Here's how the part is built. I have some questions about the finished solid (model axes, mm). Face numbers are marked on the shaded views. A direction names the side the tool comes from. Coordinates: 2 decimals unless noted, no trailing zeros. Write each loop counter-clockwise with the first axis right and the second up, starting at its lowest first coordinate (ties: lowest second). Pieces come first, ordered by that corner, then holes. Notation, with made-up numbers: (-12, 12) -> (25, 12) arc R20 cw to (25, 28) -> close; hole circle Ø9 at (58.25, 53.5). An arc over 180 degrees is marked (long way). Answer in a Markdown table with one row per item. Add a question column.
Autodesk Inventor part; units mm, degrees
ref_plane "YZ Plane" through (0, 0, 0) normal (1, 0, 0) x (0, 1, 0)
ref_plane "XZ Plane" through (0, 0, 0) normal (0, 1, 0) x (-1, 0, 0)
ref_plane "XY Plane" through (0, 0, 0) normal (0, 0, 1) x (1, 0, 0)
sketch "スケッチ1" plane through (0, 0, 0) normal (0, 0, 1) x (1, 0, 0)
  line L0 (-25, 25) -> (25, 25)
  line L1 (25, 25) -> (25, -25)
  line L2 (25, -25) -> (-25, -25)
  line L3 (-25, -25) -> (-25, 25)
  line L4 (-23, 23) -> (23, 23)
  line L5 (23, 23) -> (23, -23)
  line L6 (23, -23) -> (-23, -23)
  line L7 (-23, -23) -> (-23, 23)
  point P0 (0, 0)
  dimension "d0" = 50
  dimension "d1" = 50
  dimension "d4" = 25
  dimension "d5" = 25
  dimension "d6" = 46
  dimension "d7" = 2
  dimension "d8" = 46
  dimension "d9" = 2
extrude "押し出し1" add sketch "スケッチ1" along normal blind 50
sketch "スケッチ2" plane through (25, -25, 0) normal (1, 0, 0) x (0, 0, -1)
  line L0 (-50, 50) -> (-50, 0)
  line L1 (0, 0) -> (-50, 0)
  line L2 (-50, 20) -> (-13.5, 20)
  line L3 (-13.5, 7) -> (-50, 7)
  line L4 (-50, 7) -> (-50, 20)
  arc A0 (-13.5, 7) -> (-13.5, 20) centre (-13.5, 13.5) ccw
  point P0 (0, 25)
  point P1 (-7, 13.5)
  dimension "d34" = 13
  dimension "d35" = 7
  dimension "d43" = 13
  dimension "d44" = 6.5
  dimension "d46" = 36.5
extrude "押し出し2" cut sketch "スケッチ2" against normal blind 30.5
sketch "スケッチ3" plane through (25, -25, 0) normal (1, 0, 0) x (0, 0, -1)
  arc A0 (-13.5, 7) -> (-13.5, 20) centre (-13.5, 13.5) ccw
  line L0 (-13.5, 7) -> (-50, 7)
  circle A1 centre (-7, 21.5) radius 1
  circle A2 centre (-43, 21.5) radius 1
  circle A3 centre (-43, 5.5) radius 1
  circle A4 centre (-7, 5.5) radius 1
  point P0 (0, 25)
  dimension "d47" = 8
  dimension "d48" = 8
  dimension "d49" = 16
  dimension "d50" = 1.5
  dimension "d51" = 36
  dimension "d52" = 36
  dimension "d53" = 6.5
  dimension "d55" = 2
  dimension "d56" = 6.5
hole "穴1" at (25, -19.5, 43) at (25, -3.5, 7) at (25, -19.5, 7) at (25, -3.5, 43) direction (-1, 0, 0) diameter 2 depth 2 tip angle 118 counterbore diameter 4 counterbore depth 0.5
sketch "スケッチ11" plane through (25, -25, 0) normal (1, 0, 0) x (0, 0, -1)
  line L0 (0, 0) -> (-50, 0)
  circle A0 centre (-27.5, 37.5) radius 1.5
  line L1 (-50, 50) -> (-50, 20)
  circle A1 centre (-36.5, 13.5) radius 1.5
  line L2 (0, 50) -> (0, 0)
  point P0 (0, 25)
  dimension "d108" = 13.5
  dimension "d109" = 3
  dimension "d110" = 13.5
  dimension "d128" = 24
  dimension "d137" = 27.5
hole "穴6" at (25, -11.5, 36.5) at (25, 12.5, 27.5) direction (-1, 0, 0) diameter 4 end through all
sketch "スケッチ17" plane through (-25, 25, 50) normal (0, 1, 0) x (1, 0, 0)
  line L0 (0, 50) -> (50, 50)
  line L1 (0, 0) -> (50, 0)
  circle A0 centre (14, 40) radius 1.5
  circle A1 centre (36, 40) radius 1.5
  circle A2 centre (14, 10) radius 1.5
  circle A3 centre (36, 10) radius 1.5
  point P0 (49.5, 0)
  point P1 (49.5, 50)
  point P2 (25, 50)
  dimension "d196" = 3
  dimension "d199" = 10
  dimension "d200" = 10
  dimension "d201" = 10
  dimension "d202" = 10
  dimension "d239" = 22
  dimension "d240" = 22
  dimension "d241" = 11
  dimension "d242" = 11
hole "穴12" at (11, 25, 40) at (-11, 25, 40) at (11, 25, 10) at (-11, 25, 10) direction (0, -1, 0) diameter 3 depth 2 tip angle 118
thread "ねじ1"
thread "ねじ2"
thread "ねじ3"
thread "ねじ4"
properties part number "05" material "アルミニウム 6061"
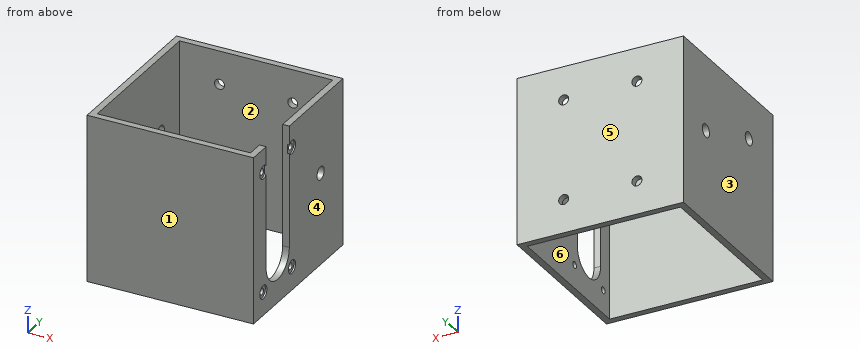
Q1. Imagine slicing it at B-B on y = -3.5. Please give me the cut outline in (x, z), plus the area to 3 significant figures.
Q2. Imagine slicing it at A-A on x = -3.5. Please give me the cut outline in (y, z), plus the area to 3 significant figures.
Q3. If we mould it in two halves opening along X, with no side actions, what happens to the marked faces 1, 2, 3 and 4? For each: pulls with the +X half, pulls with the -X half, needs draft (parallel to the pull), parting line crosses it, or undercut.
Q4. For the marked faces 5 and 6, which set-ups out of +Z, -Z, +X, -X, +Y, -Y let a thin tool reach every point of the face, with its end or its side?
Q5. I need wall thicknesses on line 1 (Z direction, x = -11, y = 23.5); line 2 (Z direction, x = 24.85, y = -19.5); line 3 (X direction, y = 24, z = 10). Which ranges of each line are inside material? Lowest first, please. Write a range as [from, to].
Q6. Imagine slicing it at D-D on z = 40. Please give me the cut outline in (x, y).
Q7. I'm going to push a flat-ended pin straight in: P1, Ø1.8, axis at x = 11, z = 10, coming from the +Y side. Where does the tip first touch, or does it pass through?
Q8. Imagine slicing it at C-C on x = 11. Please give me the cut outline in (y, z).
Result sheet:
| question | item | result |
|---|---|---|
| 1 | outline | (-25, 0) -> (-23, 0) -> (-23, 50) -> (-25, 50) -> close; (23, 0) -> (25, 0) -> (25, 5) -> (24.5, 5) -> (24.5, 6) -> (23, 6) -> close; (23, 8) -> (24.5, 8) -> (24.5, 9) -> (25, 9) -> (25, 41) -> (24.5, 41) -> (24.5, 42) -> (23, 42) -> close; (23, 44) -> (24.5, 44) -> (24.5, 45) -> (25, 45) -> (25, 50) -> (23, 50) -> close |
| 1 | area | 190 mm^2 |
| 2 | outline | (-25, 0) -> (-23, 0) -> (-23, 50) -> (-25, 50) -> close; (23, 0) -> (25, 0) -> (25, 50) -> (23, 50) -> close |
| 2 | area | 200 mm^2 |
| 3 | face 1 | needs draft |
| 3 | face 2 | undercut |
| 3 | face 3 | pulls with the -X half |
| 3 | face 4 | pulls with the +X half |
| 4 | face 5 | +Z, -Z, +X, -X, +Y |
| 4 | face 6 | +Z, -Z |
| 5 | line 1 | z = [0, 8.5], [11.5, 38.5], [41.5, 50] |
| 5 | line 2 | z = [0, 5], [9, 41], [45, 50] |
| 5 | line 3 | x = [-25, -12.5], [-9.5, 9.5], [12.5, 25] |
| 6 | outline | (-25, -25) -> (25, -25) -> (25, -18) -> (23, -18) -> (23, -23) -> (-23, -23) -> (-23, 23) -> (-12.5, 23) -> (-12.5, 25) -> (-25, 25) -> close; (-9.5, 23) -> (9.5, 23) -> (9.5, 25) -> (-9.5, 25) -> close; (12.5, 23) -> (23, 23) -> (23, -5) -> (25, -5) -> (25, 25) -> (12.5, 25) -> close |
| 7 | P1 | stops at y = -23 |
| 8 | outline | (-25, 0) -> (-23, 0) -> (-23, 50) -> (-25, 50) -> close; (23, 0) -> (25, 0) -> (25, 8.5) -> (23, 8.5) -> close; (23, 11.5) -> (25, 11.5) -> (25, 38.5) -> (23, 38.5) -> close; (23, 41.5) -> (25, 41.5) -> (25, 50) -> (23, 50) -> close |
